Work out the finished part from the listing and answer in its coordinate system (mm). Face numbers are marked on the shaded views. A direction names the side the tool comes from. Give positions to 0.01 mm unless a question says otherwise; leave off trailing zeros. Order: outer loops, then holes, each group sorted by start corner. A loop starts at its lowest first (then second) coordinate and runs counter-clockwise, first axis right, second up. Notation, with made-up numbers: (71, 34) -> (124, 34) arc R22 cw to (124, 58) -> close; hole circle Ø2 at (-18, 47.25). An arc over 180 degrees is marked (long way). Answer as CSV lines item,"result". Start each with the question number.
1. Flat-ended cylindrical pins translate along their axes: pin 1 (2 mm diameter, centred on x = -1, y = 3, fed in from +Z); pin 2 (1.2 mm diameter, centred on y = -1, z = 75, fed in from +X); pin 3 (1.2 mm diameter, centred on x = 3, y = -1.5, fed in from -Z). Find the tip coordinate at first contact, or state that the pin passes through.
2. A cutting plane is placed at C-C (x = -0.75). Give the vertices of the cut face in (y, z).
3. Find the intervals of material crossed by L1, parallel to Z at x = -3.45, y = 0; L2, parallel to Y at x = -3.25, z = 77.5; L3, parallel to Z at x = -1.75, y = -0.25, in increasing order.
4. For the marked faces 1 and 2, determine the directions among +Z, -Z, +X, -X, +Y, -Y from which every point of the face is accessible in a straight line to the end or side of a thin tool.
5. A cutting plane is placed at B-B (z = 23). Give the vertices of the cut face in (x, y), then the cut area to 3 significant figures.
6. A cutting plane is placed at A-A (y = 0). Give the vertices of the cut face in (x, z).
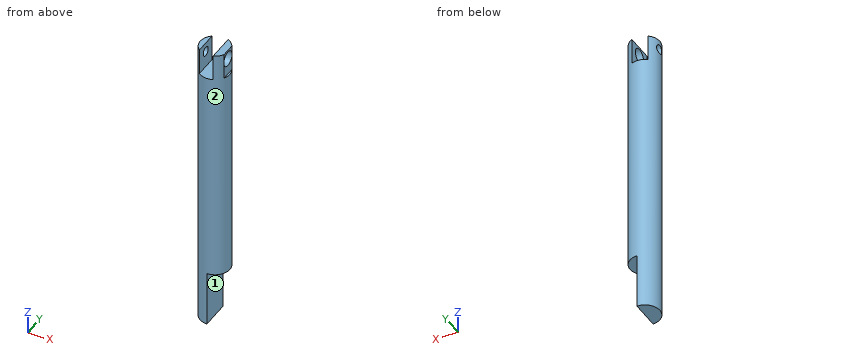
Autodesk Inventor part; units mm, degrees
ref_plane "YZ Plane" through (0, 0, 0) normal (1, 0, 0) x (0, 1, 0)
ref_plane "XZ Plane" through (0, 0, 0) normal (0, 1, 0) x (-1, 0, 0)
ref_plane "XY Plane" through (0, 0, 0) normal (0, 0, 1) x (1, 0, 0)
sketch "Sketch1" plane through (0, 0, 0) normal (0, 0, 1) x (1, 0, 0)
  circle A0 centre (0, 0) radius 4
  dimension "d0" = 8
extrude "Extrusion1" add sketch "Sketch1" along normal blind 80
sketch "Sketch2" plane through (0, 0, 0) normal (0, 1, 0) x (-1, 0, 0)
  line L0 (0, 0) -> (-5.3393, 0)
  line L1 (-5.3393, 0) -> (-5.3393, 15)
  line L2 (-5.3393, 15) -> (0, 15)
  line L3 (0, 15) -> (0, 0)
  line L4 (2.5, 80) -> (-1.5, 80)
  line L5 (-1.5, 80) -> (-1.5, 73)
  line L6 (-1.5, 73) -> (2.5, 73)
  line L7 (2.5, 73) -> (2.5, 80)
  line L8 (4, 80) -> (-4, 80) construction
  line L9 (-4, 80) -> (-3.5, 80)
  line L10 (-3.5, 80) -> (-3.5, 73)
  line L11 (-3.5, 73) -> (-4, 73)
  line L12 (-4, 73) -> (-4, 80)
  point P0 (-3.75, 73)
  dimension "d3" = 4
  dimension "d4" = 7
  dimension "d5" = 2.5
  dimension "d6" = 15
  dimension "d9" = 2
extrude "Extrusion2" cut sketch "Sketch2" along normal through all both and the other way through all
sketch "Sketch3" plane through (3.5, -1.9365, 73) normal (1, 0, 0) x (0, 0, -1)
  circle A0 centre (-4.5, 1.9365) radius 1.5
  line L0 (-7, 0) -> (-7, 3.873)
  point P0 (73, 1.9365)
  point P1 (-7, 1.9365)
  dimension "d10" = 3
  dimension "d11" = 2.5
hole "Hole1" at (3.5, 0, 77.5) direction (-1, 0, 0) diameter 2.459 end through all counterbore diameter 4 counterbore depth 3
properties part number "Servo_Strut_CPY_CPY"
Answer sheet:
1,pin 1,"stops at z = 73"
1,pin 2,"stops at x = 3.5"
1,pin 3,"stops at z = 15"
2,outline,"(-3.93, 0) -> (3.93, 0) -> (3.93, 73) -> (-3.93, 73) -> close"
3,L1,"z = 0 to 76.27, 78.73 to 80"
3,L2,"y = -2.33 to -1.23, 1.23 to 2.33"
3,L3,"z = 0 to 73"
4,face 1,"-Z, +X, +Y, -Y"
4,face 2,"+Z, -Z"
5,outline,"circle Ø8 at (0, 0)"
5,area,"50.3 mm^2"
6,outline,"(-4, 0) -> (0, 0) -> (0, 15) -> (4, 15) -> (4, 73) -> (3.5, 73) -> (3.5, 75.5) -> (1.5, 75.5) -> (1.5, 73) -> (-2.5, 73) -> (-2.5, 76.27) -> (-4, 76.27) -> close; (-4, 78.73) -> (-2.5, 78.73) -> (-2.5, 80) -> (-4, 80) -> close; (1.5, 79.5) -> (3.5, 79.5) -> (3.5, 80) -> (1.5, 80) -> close"
